from build123d import *

# Parameters (mm, degrees)
SKETCH2_R           = 1.905
BOSS_EXTRUDE1_DEPTH = 4.7625


with BuildPart() as part:
    # Sketch2 → Boss-Extrude1 (new body)
    with BuildSketch(Plane.XY):
        with BuildLine():
            Line((-19.404343504, -3.787653884), (-2.894343504, -3.787653884))
            ThreePointArc((-2.894343504, -3.787653884), (-1.996317892, -3.415679496), (-1.624343504, -2.517653884))
            Line((-1.624343504, -2.517653884), (-1.624343504, 13.992346116))
            ThreePointArc((-1.624343504, 13.992346116), (-1.996317892, 14.890371728), (-2.894343504, 15.262346116))
            Line((-2.894343504, 15.262346116), (-19.404343504, 15.262346116))
            ThreePointArc((-19.404343504, 15.262346116), (-20.302369116, 14.890371728), (-20.674343504, 13.992346116))
            Line((-20.674343504, 13.992346116), (-20.674343504, -2.517653884))
            ThreePointArc((-20.674343504, -2.517653884), (-20.302369116, -3.415679496), (-19.404343504, -3.787653884))
        make_face()
        with Locations((-17.005652309, 11.593654921)):
            Circle(SKETCH2_R, mode=Mode.SUBTRACT)
        with Locations((-5.2930347, 11.593654921)):
            Circle(SKETCH2_R, mode=Mode.SUBTRACT)
        with Locations((-5.2930347, -0.118962689)):
            Circle(SKETCH2_R, mode=Mode.SUBTRACT)
        with Locations((-17.005652309, -0.118962689)):
            Circle(SKETCH2_R, mode=Mode.SUBTRACT)
        with BuildLine():
            Line((-12.673343504, 7.769346116), (-9.625343504, 7.769346116))
            ThreePointArc((-9.625343504, 7.769346116), (-11.149343504, 3.197346116), (-12.673343504, 7.769346116))
        make_face(mode=Mode.SUBTRACT)
    extrude(amount=BOSS_EXTRUDE1_DEPTH)


solid = part.part
Verification items for the finished model (mm, model axes). A direction names the side the tool comes from. Coordinates: 2 decimals unless noted, no trailing zeros. Order: outer loops, then holes, each group sorted by start corner. A loop starts at its lowest first (then second) coordinate and runs counter-clockwise, first axis right, second up. Notation, with made-up numbers: (33, -30) -> (82, -30) arc R12 ccw to (82, -17) -> close; hole circle Ø5 at (-39, 74). An arc over 180 degrees is marked (long way). Put each result on its own line as item: value. Start each with the question number.
1. Go/stop test with flat-tipped pins: pin 1 Ø3 at (x, y) = (-17.01, 11.59) entering from -Z; pin 2 Ø8 at (x, y) = (-10, -0.5) entering from -Z. Record where each tip stops, or that it passes through.
2. Cross-section at A-A, the plane y = 10.75. Record the boundary of the cut face in (x, z).
3. Cross-section at C-C, the plane z = 4.35. Record the boundary of the cut face in (x, y) (3 decimals), then the cut area to 3 significant figures.
4. Cross-section at B-B, the plane x = -13. Record the boundary of the cut face in (y, z), then the cut area to 3 significant figures.
5. Access from +Z, -Z, +X, -X, +Y, -Y to the whole of each face (thin tool, end or side, straight path). Record for faces 1 (the cylindrical face through (-20.29, 14.9, 2.35)), 2 (the flat face through (-11, 7.769, 2)).
6. Mould release check, pull along X, two halves, no side actions. Record for faces 3 (the flat face through (-11, 8, 4.762)), 4 (the cylindrical face through (-15.246, -0.849, 2.348)), 5 (the cylindrical face through (-20.31, -3.41, 2.35)): released by +X, released by -X, zero draft, split by the parting line, or undercut.
7. Material ranges on L1, parallel to X at y = 0.25, z = 1.3; L2, parallel to Y at x = -17, z = 4.5; L3, parallel to X at y = 10.5, z = 4.5, recorded low to high. Write a range as [from, to].
8. Cross-section at D-D, the plane x = -5.5. Record the boundary of the cut face in (y, z), then the cut area to 3 significant figures.
Computed:
1. pin 1: through
1. pin 2: z = 0
2. outline: (-20.67, 0) -> (-18.71, 0) -> (-18.71, 4.76) -> (-20.67, 4.76) -> close; (-15.3, 0) -> (-7, 0) -> (-7, 4.76) -> (-15.3, 4.76) -> close; (-3.59, 0) -> (-1.62, 0) -> (-1.62, 4.76) -> (-3.59, 4.76) -> close
3. outline: (-20.674, -2.518) arc R1.27 ccw to (-19.404, -3.788) -> (-2.894, -3.788) arc R1.27 ccw to (-1.624, -2.518) -> (-1.624, 13.992) arc R1.27 ccw to (-2.894, 15.262) -> (-19.404, 15.262) arc R1.27 ccw to (-20.674, 13.992) -> close; hole circle Ø3.81 at (-17.006, -0.119); hole circle Ø3.81 at (-17.006, 11.594); hole (-12.673, 7.769) arc R2.54 ccw (long way) to (-9.625, 7.769) -> close; hole circle Ø3.81 at (-5.293, -0.119); hole circle Ø3.81 at (-5.293, 11.594)
3. area: 297 mm2
4. outline: (-3.79, 0) -> (4, 0) -> (4, 4.76) -> (-3.79, 4.76) -> close; (7.48, 0) -> (15.26, 0) -> (15.26, 4.76) -> (7.48, 4.76) -> close
4. area: 74.2 mm2
5. face 1: +Z, -Z, -X, +Y
5. face 2: +Z, -Z
6. face 3: zero draft
6. face 4: undercut
6. face 5: released by -X
7. L1: [-20.67, -18.87], [-15.14, -7.16], [-3.42, -1.62]
7. L2: [-3.79, -2.02], [1.79, 9.69], [13.5, 15.26]
7. L3: [-20.67, -18.57], [-15.45, -6.85], [-3.73, -1.62]
8. outline: (-3.79, 0) -> (-2.01, 0) -> (-2.01, 4.76) -> (-3.79, 4.76) -> close; (1.77, 0) -> (9.7, 0) -> (9.7, 4.76) -> (1.77, 4.76) -> close; (13.49, 0) -> (15.26, 0) -> (15.26, 4.76) -> (13.49, 4.76) -> close
8. area: 54.7 mm2
